Geometry: final body of the model. Coordinates: model frame, mm. A direction names the side the tool comes from. Round coordinates to 2 decimals unless told otherwise and drop trailing zeros. Write each loop counter-clockwise with the first axis right and the second up, starting at its lowest first coordinate (ties: lowest second). Pieces come first, ordered by that corner, then holes. Notation, with made-up numbers: (63, 77) - (100, 77) arc R32 cw to (100, 110) - close; hole circle Ø5 at (59.5, -15.75). An arc over 180 degrees is marked (long way). Use a Markdown table: item, result. Add a question column.
```python
from build123d import *

# Parameters (mm, degrees)
F0_W     = 34.29
F0_H     = 63.5
F1_DEPTH = 25.4


with BuildPart() as f1:
    # F0 (on Top) → F1 (new body)
    with BuildSketch(Plane.XY):
        with Locations((6.322508, 33.528001)):
            Rectangle(F0_W, F0_H)
        Polygon((19.022508, 7.366001), (6.322508, 7.366001), (-6.377492, 7.366001), (-6.377492, 9.271001), (5.6515, 9.271001), (19.022508, 9.271001), align=None, mode=Mode.SUBTRACT)
        Polygon((19.022508, 12.700001), (6.322508, 12.700001), (-6.377492, 12.700001), (-6.377492, 14.605001), (7.876809, 14.605001), (19.022508, 14.605001), align=None, mode=Mode.SUBTRACT)
        Polygon((19.022508, 18.034001), (6.322508, 18.034001), (-6.377492, 18.034001), (-6.377492, 19.939001), (5.6515, 19.939001), (19.022508, 19.939001), align=None, mode=Mode.SUBTRACT)
        Polygon((19.022508, 23.368001), (6.322508, 23.368001), (-6.377492, 23.368001), (-6.377492, 25.273001), (5.6515, 25.273001), (19.022508, 25.273001), align=None, mode=Mode.SUBTRACT)
        Polygon((19.022508, 28.702001), (6.322508, 28.702001), (-6.377492, 28.702001), (-6.377492, 30.607001), (5.6515, 30.607001), (19.022508, 30.607001), align=None, mode=Mode.SUBTRACT)
        Polygon((19.022508, 60.706001), (6.322508, 60.706001), (-6.377492, 60.706001), (-6.377492, 62.611001), (5.6515, 62.611001), (19.022508, 62.611001), align=None, mode=Mode.SUBTRACT)
        Polygon((19.022508, 34.036001), (6.322508, 34.036001), (-6.377492, 34.036001), (-6.377492, 35.941001), (5.6515, 35.941001), (19.022508, 35.941001), align=None, mode=Mode.SUBTRACT)
        Polygon((19.022508, 39.370001), (6.322508, 39.370001), (-6.377492, 39.370001), (-6.377492, 41.275001), (5.6515, 41.275001), (19.022508, 41.275001), align=None, mode=Mode.SUBTRACT)
        Polygon((19.022508, 44.704001), (6.322508, 44.704001), (-6.377492, 44.704001), (-6.377492, 46.609001), (5.6515, 46.609001), (19.022508, 46.609001), align=None, mode=Mode.SUBTRACT)
        Polygon((19.022508, 50.038001), (6.322508, 50.038001), (-6.377492, 50.038001), (-6.377492, 51.943001), (5.6515, 51.943001), (19.022508, 51.943001), align=None, mode=Mode.SUBTRACT)
        Polygon((19.022508, 55.372001), (6.322508, 55.372001), (-6.377492, 55.372001), (-6.377492, 57.277001), (5.6515, 57.277001), (19.022508, 57.277001), align=None, mode=Mode.SUBTRACT)
    extrude(amount=F1_DEPTH)


solid = f1.part
```
1) Draft query along Y for faces 3 (the flat face through (6, 27, 0)), 4 (the flat face through (19.023, 8, 13)). Return one class per face: released by +Y, released by -Y, zero draft, split by the parting line, or undercut.
2) Section A-A, the plane y = 51. Return the cut outline in (x, z), then the cut area to 3 significant figures.
3) Section B-B, the plane x = 0.5. State how many separate pieces and enclosed holes the cut face has, then the cut area to 3 significant figures.
4) Material intervals for L1, parallel to X at y = 29, z = 14, sorted ascending. Write a range as from..to.
5) Set-up query: faces 1 (the flat face through (23.468, 33, 13)), 2 (the flat face through (7, 18.034, 13)). Return all of +Z, -Z, +X, -X, +Y, -Y with unobstructed straight access to the full face (end or side cutting, diameter ignored); none if empty.
Output values:
| question | item | result |
|---|---|---|
| 1 | face 3 | zero draft |
| 1 | face 4 | undercut |
| 2 | outline | (-10.82, 0) - (-6.38, 0) - (-6.38, 25.4) - (-10.82, 25.4) - close; (19.02, 0) - (23.47, 0) - (23.47, 25.4) - (19.02, 25.4) - close |
| 2 | area | 226 mm^2 |
| 3 | separate pieces | 12 |
| 3 | enclosed holes | 0 |
| 3 | area | 1,080 mm^2 |
| 4 | L1 | x = -10.82..-6.38, 19.02..23.47 |
| 5 | face 1 | +Z, -Z, +X, +Y, -Y |
| 5 | face 2 | +Z, -Z |
